from build123d import *

# Parameters (mm, degrees)
SKETCH1_R           = 13.5
BOSS_EXTRUDE1_DEPTH = 67
SKETCH2_R           = 11.5
BOSS_EXTRUDE2_DEPTH = 16
SKETCH3_R           = 9.5
BOSS_EXTRUDE3_DEPTH = 9
SKETCH4_R           = 7.5
BOSS_EXTRUDE4_DEPTH = 16
CUT_EXTRUDE1_DEPTH  = 111.847868721
SKETCH7_R           = 2.5
CUT_EXTRUDE2_DEPTH  = 1.27


with BuildPart() as part:
    # Sketch1 → Boss-Extrude1 (new body)
    with BuildSketch(Plane(origin=(0, 0, 0), x_dir=(1, 0, 0), z_dir=(0, 1, 0))):
        with Locations(Location((0, 0, 0), (0, 0, 270))):
            Circle(SKETCH1_R)
    extrude(amount=BOSS_EXTRUDE1_DEPTH)

    # Sketch2 → Boss-Extrude2 (add)
    with BuildSketch(Plane(origin=(0, 67, 0), x_dir=(1, 0, 0), z_dir=(0, 1, 0))):
        with Locations(Location((0, 0, 0), (0, 0, 270))):
            Circle(SKETCH2_R)
    extrude(amount=BOSS_EXTRUDE2_DEPTH)

    # Sketch3 → Boss-Extrude3 (add)
    with BuildSketch(Plane(origin=(0, 83, 0), x_dir=(1, 0, 0), z_dir=(0, 1, 0))):
        with Locations(Location((0, 0, 0), (0, 0, 270))):
            Circle(SKETCH3_R)
    extrude(amount=BOSS_EXTRUDE3_DEPTH)

    # Sketch4 → Boss-Extrude4 (add)
    with BuildSketch(Plane(origin=(0, 92, 0), x_dir=(1, 0, 0), z_dir=(0, 1, 0))):
        with Locations(Location((0, 0, 0), (0, 0, 270))):
            Circle(SKETCH4_R)
    extrude(amount=BOSS_EXTRUDE4_DEPTH)

    # Sketch6 → Cut-Extrude1 (cut, through all)
    with BuildSketch(Plane(origin=(7.5, 0, 0), x_dir=(0, 0, -1), z_dir=(1, 0, 0))):
        Polygon((-7.319182821, 108), (8.150119574, 104), (7.994537509, 108), align=None)
    extrude(amount=-CUT_EXTRUDE1_DEPTH, mode=Mode.SUBTRACT)

    # Sketch7 → Cut-Extrude2 (cut)
    with BuildSketch(Plane.XY.offset(7.5)):
        with Locations((0, 104.6)):
            Circle(SKETCH7_R)
    extrude(amount=-CUT_EXTRUDE2_DEPTH, mode=Mode.SUBTRACT)


solid = part.part
Read the model definition and answer for the solid it produces. Units are mm, in the model's axes. A direction names the side the tool comes from. Coordinates: 2 decimals unless noted, no trailing zeros. Loops run counter-clockwise (first coordinate to the right, second up) from the corner with the lowest first, then second, coordinate; pieces in that order, holes last. Notation, with made-up numbers: (10.25, 13) -> (34.25, 13) arc R24 cw to (34.25, 40) -> close; hole circle Ø6 at (-17, -34). An arc over 180 degrees is marked (long way). Write item = value, one per line. Start each with the question number.
1) The part is cut by section D-D, the plane z = -5.75. Determine the outline of the cut face in (x, y), plus the area to 3 significant figures.
2) Find the intervals of material crossed by L1, parallel to Z at x = -0.25, y = 69; L2, parallel to Y at x = 0, z = 6.75; L3, parallel to Y at x = -2, z = -8.25, in increasing order. Write a range as from..to.
3) Given P1, Ø12, axis at x = -3.5, y = 20.5, coming from the +Z side; P2, Ø12, axis at x = 0, z = -9, coming from the +Y side; P3, Ø5, axis at x = 9.5, y = 75, coming from the +Z side; P4, Ø2, axis at y = 79, z = 9.5, coming from the +X side, each flat-ended and moving along its own axis, determine where each tip first touches the part or whether it passes through.
4) The part is cut by section C-C, the plane y = 100. Determine the outline of the cut face in (x, z), plus the area to 3 significant figures.
5) For faces 1 (the face through (0.11, 106.11, 0.01)), 2 (the face through (-5.78, 87.44, -7.54)), determine the directions among +Z, -Z, +X, -X, +Y, -Y from which every point of the face is accessible in a straight line to the end or side of a thin tool.
6) The mould has two halves that part along Y. Classify faces 3 (the face through (-2.5, 104.7, 6.7)), 4 (the face through (0, 105, 6.23)), 5 (the face through (-13.18, 33.03, -2.93)), 6 (the face through (8, 92, 1)): pulls with the +Y half, pulls with the -Y half, needs draft (parallel to the pull), parting line crosses it, or undercut.
7) The part is cut by section B-B, the plane z = -10.5. Determine the outline of the cut face in (x, y), plus the area to 3 significant figures.
8) The part is cut by section A-A, the plane x = 0. Determine the outline of the cut face in (y, z), plus the area to 3 significant figures.
Result:
q1.outline = (-12.21, 0) -> (12.21, 0) -> (12.21, 67) -> (9.96, 67) -> (9.96, 83) -> (7.56, 83) -> (7.56, 92) -> (4.82, 92) -> (4.82, 104.62) -> (-4.82, 104.62) -> (-4.82, 92) -> (-7.56, 92) -> (-7.56, 83) -> (-9.96, 83) -> (-9.96, 67) -> (-12.21, 67) -> close
q1.area = 2,210 mm²
q2.L1 = -11.5..11.5
q2.L2 = 0..102.1, 107.1..107.85
q2.L3 = 0..92
q3.P1 = 13.5
q3.P2 = 105.33
q3.P3 = 9.12
q3.P4 = 7.75
q4.outline = circle Ø15 at (0, 0)
q4.area = 177 mm²
q5.face_1 = -Z, +X, -X, +Y
q5.face_2 = +Y
q6.face_3 = undercut
q6.face_4 = undercut
q6.face_5 = needs draft
q6.face_6 = pulls with the +Y half
q7.outline = (-8.49, 0) -> (8.49, 0) -> (8.49, 67) -> (4.69, 67) -> (4.69, 83) -> (-4.69, 83) -> (-4.69, 67) -> (-8.49, 67) -> close
q7.area = 1,290 mm²
q8.outline = (0, -13.5) -> (67, -13.5) -> (67, -11.5) -> (83, -11.5) -> (83, -9.5) -> (92, -9.5) -> (92, -7.5) -> (104.17, -7.5) -> (108, 7.32) -> (108, 7.5) -> (107.1, 7.5) -> (107.1, 6.23) -> (102.1, 6.23) -> (102.1, 7.5) -> (92, 7.5) -> (92, 9.5) -> (83, 9.5) -> (83, 11.5) -> (67, 11.5) -> (67, 13.5) -> (0, 13.5) -> close
q8.area = 2,550 mm²
